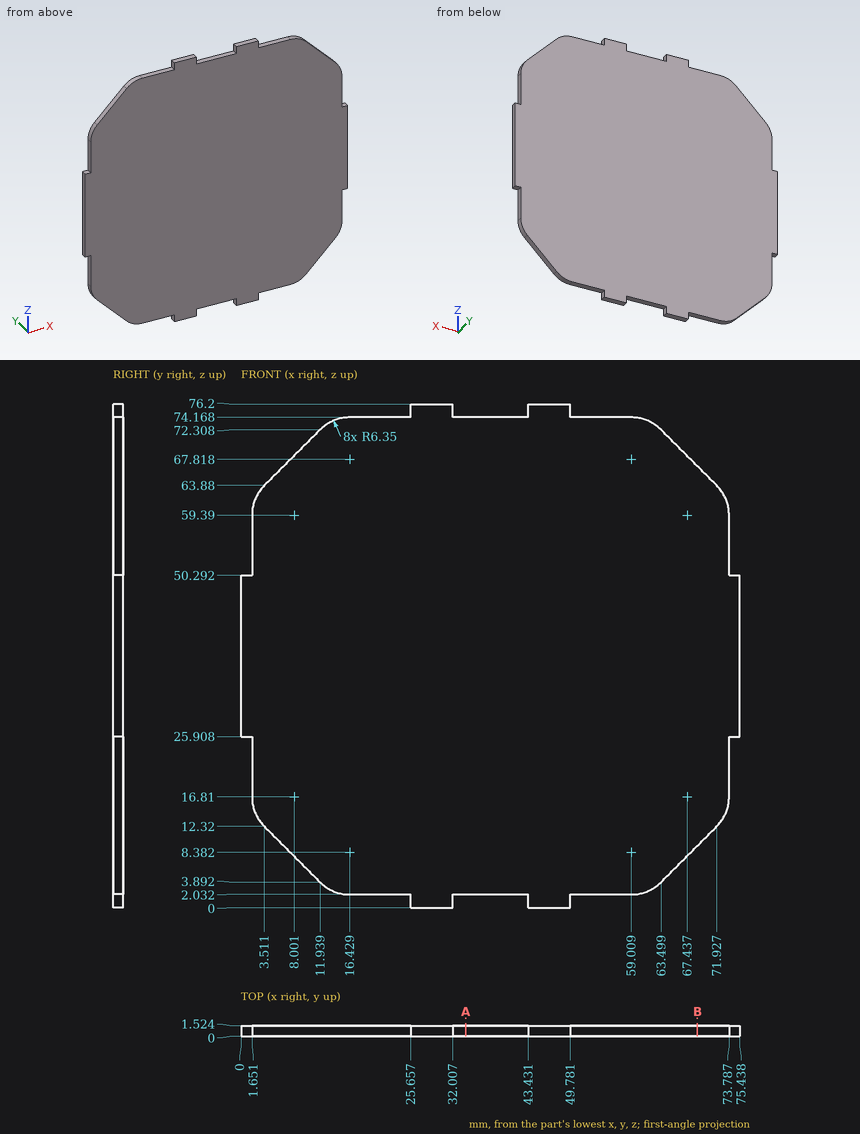
For this review, use the dimensioned drawing (mm, ordinates from the lowest corner) and the shaded views. Coordinates: 2 decimals unless noted, no trailing zeros. Loops run counter-clockwise (first coordinate to the right, second up) from the corner with the lowest first, then second, coordinate; pieces in that order, holes last. Notation, with made-up numbers: (-1, 76.5) -> (39, 76.5) arc R6 ccw to (39, 85.5) -> close; hole circle Ø3 at (-32, 48). An arc over 180 degrees is marked (long way). Use a Markdown table: item, result. Add a question column.
1. Add section B-B on x = 69. Write out the cut boundary in (y, z).
2. Clearance check with flat-ended pins moving along their axes: pin 1 Ø0.8 at (y, z) = (1, 75) entering from +X; pin 2 Ø0.8 at (y, z) = (0.5, 75.5) entering from -X; pin 3 Ø0.5 at (x, y) = (53.5, 0.5) entering from -Z. State where each tip first meets the part, or that it passes through.
3. To check wall thickness, follow line 1 (Z direction, x = 56.5, y = 0.75); line 2 (X direction, y = 1.15, z = 18); line 3 (Z direction, x = 59.5, y = 1.3). State the ranges of each line that lie inside material, in increasing order.
4. Add section A-A on x = 34. Write out the cut boundary in (y, z).
Returned:
| question | item | result |
|---|---|---|
| 1 | outline | (0, 9.39) -> (1.52, 9.39) -> (1.52, 66.81) -> (0, 66.81) -> close |
| 2 | pin 1 | stops at x = 49.78 |
| 2 | pin 2 | stops at x = 25.66 |
| 2 | pin 3 | stops at z = 2.03 |
| 3 | line 1 | z = 2.03 to 74.17 |
| 3 | line 2 | x = 1.65 to 73.79 |
| 3 | line 3 | z = 2.05 to 74.15 |
| 4 | outline | (0, 2.03) -> (1.52, 2.03) -> (1.52, 74.17) -> (0, 74.17) -> close |
